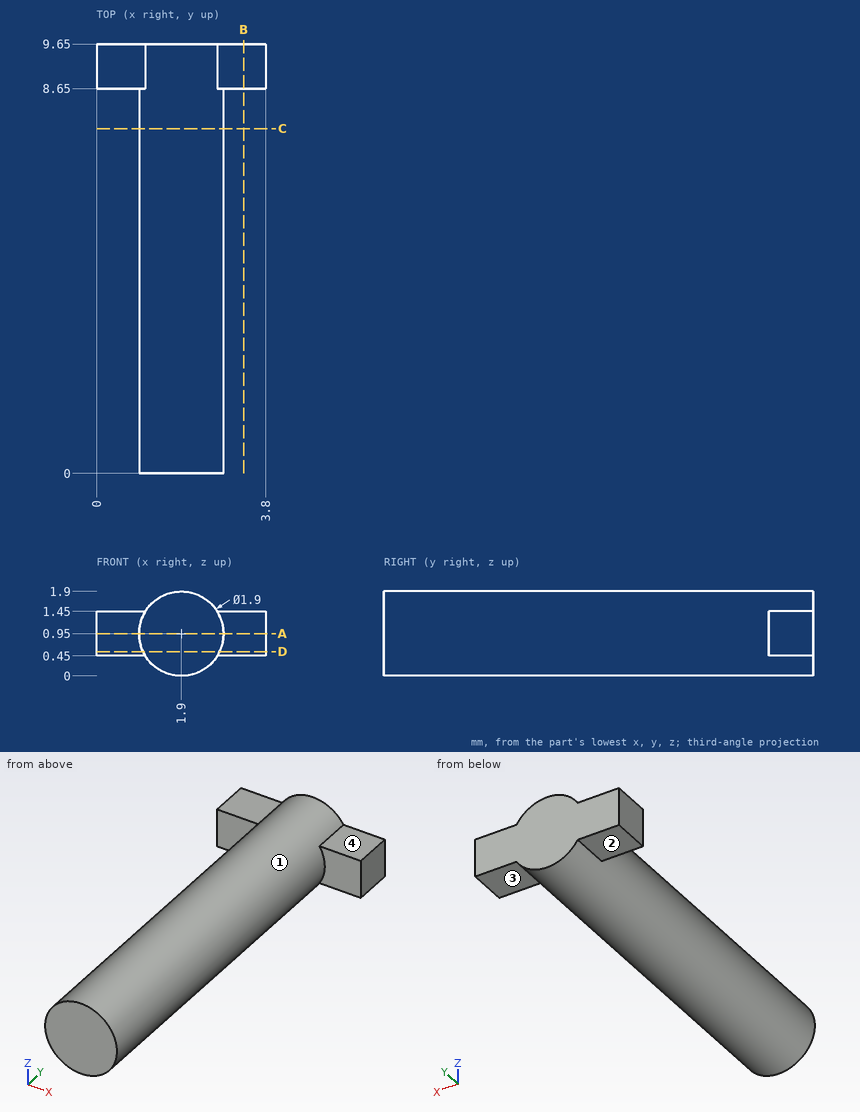
Study the drawing (mm; zero at the part's minimum x, y, z) and answer. A direction names the side the tool comes from. Coordinates: 2 decimals unless noted, no trailing zeros. Order: outer loops, then holes, each group sorted by start corner. A loop starts at its lowest first (then second) coordinate and runs counter-clockwise, first axis right, second up. Notation, with made-up numbers: M 85,55.5 L 89,55.5 A16 cw 89,84.5 Z; hole C -0.75,78 d3. An arc over 180 degrees is marked long. Use CSV: the item, a comma, the result in double quotes.
Q1. Section D-D (z = 0.55) is taken. Determine the outline of the cut face in (x, y), then the cut area to 3 significant figures.
Here are the results:
outline,"M 0,8.65 L 1.04,8.65 L 1.04,0 L 2.76,0 L 2.76,8.65 L 3.8,8.65 L 3.8,9.65 L 0,9.65 Z"
area,"18.7 mm2"
Q2. Section A-A (z = 0.95) is taken. Determine the outline of the cut face in (x, y), then the cut area to 3 significant figures.
Here are the results:
outline,"M 0,8.65 L 0.95,8.65 L 0.95,0 L 2.85,0 L 2.85,8.65 L 3.8,8.65 L 3.8,9.65 L 0,9.65 Z"
area,"20.2 mm2"
Q3. Straight lines are drawn through the part: L1, parallel to Y at x = 3.1, z = 1.25; L2, parallel to X at y = 8.25, z = 1; L3, parallel to Z at x = 1.95, y = 9. For each, find the intervals that lie inside material, in ascending order.
Here are the results:
L1,"8.65 to 9.65"
L2,"0.95 to 2.85"
L3,"0 to 1.9"
Q4. Section B-B (x = 3.3) is taken. Determine the outline of the cut face in (y, z), then the cut area to 3 significant figures.
Here are the results:
outline,"M 8.65,0.45 L 9.65,0.45 L 9.65,1.45 L 8.65,1.45 Z"
area,"1.00 mm2"
Q5. A tool of negligible diameter and unlimited length cuts with its end or side. For the marked faces 1, 2, 3 and 4, from which of +Z, -Z, +X, -X, +Y, -Y can it reach the whole face along a straight path? Write none if from no direction.
Here are the results:
face 1,"-Y"
face 2,"-Z, -X, +Y, -Y"
face 3,"-Z, +X, +Y, -Y"
face 4,"+Z, +X, +Y, -Y"
Q6. Section C-C (y = 7.75) is taken. Determine the outline of the cut face in (x, z), then the cut area to 3 significant figures.
Here are the results:
outline,"C 1.9,0.95 d1.9"
area,"2.84 mm2"
Q7. Given pin 1 Ø1.1 at (x, y) = (0.5, 9.5) entering from +Z; pin 2 Ø1 at (x, y) = (1, 4.5) entering from -Z; pin 3 Ø1.1 at (x, y) = (0.5, 9) entering from -Z, each flat-ended and moving along its own axis, determine where each tip first touches the part or whether it passes through.
Here are the results:
pin 1,"z = 1.45"
pin 2,"z = 0.09"
pin 3,"z = 0.45"
